from build123d import *

# Parameters (mm, degrees)
F1_DEPTH = 254
F0_W     = 9.525
F0_H     = 9.525
F2_DEPTH = 228.6
F0_W_2   = 114.3
F0_H_2   = 114.3
F3_DEPTH = 177.8
F0_W_3   = 127
F0_H_3   = 127
F4_DEPTH = 127


with BuildPart() as f1:
    # F0 (on Top) → F1 (new body)
    with BuildSketch(Plane.XY):
        Polygon((28.575, 38.1), (-28.575, 38.1), (-28.575, 28.575), (-38.1, 28.575), (-38.1, -28.575), (-28.575, -28.575), (-28.575, -38.1), (28.575, -38.1), (28.575, -28.575), (38.1, -28.575), (38.1, 28.575), (28.575, 28.575), align=None)
    extrude(amount=F1_DEPTH)

    # F0 (on Top) → F2 (join)
    with BuildSketch(Plane.XY):
        Polygon((-38.1, 28.575), (-38.1, 38.1), (-28.575, 38.1), (-28.575, 47.625), (-47.625, 47.625), (-47.625, 28.575), align=None)
        with Locations((-33.3375, 33.3375)):
            Rectangle(F0_W, F0_H)
        Polygon((-38.1, -38.1), (-38.1, -28.575), (-47.625, -28.575), (-47.625, -47.625), (-28.575, -47.625), (-28.575, -38.1), align=None)
        with Locations((-33.3375, -33.3375)):
            Rectangle(F0_W, F0_H)
        Polygon((47.625, -28.575), (38.1, -28.575), (38.1, -38.1), (28.575, -38.1), (28.575, -47.625), (47.625, -47.625), align=None)
        with Locations((33.3375, -33.3375)):
            Rectangle(F0_W, F0_H)
        Polygon((28.575, 47.625), (28.575, 38.1), (38.1, 38.1), (38.1, 28.575), (47.625, 28.575), (47.625, 47.625), align=None)
        with Locations((33.3375, 33.3375)):
            Rectangle(F0_W, F0_H)
    extrude(amount=F2_DEPTH)

    # F0 (on Top) → F3 (join)
    with BuildSketch(Plane.XY):
        Rectangle(F0_W_2, F0_H_2)
        Polygon((-28.575, 47.625), (-28.575, 38.1), (28.575, 38.1), (28.575, 47.625), (47.625, 47.625), (47.625, 28.575), (38.1, 28.575), (38.1, -28.575), (47.625, -28.575), (47.625, -47.625), (28.575, -47.625), (28.575, -38.1), (-28.575, -38.1), (-28.575, -47.625), (-47.625, -47.625), (-47.625, -28.575), (-38.1, -28.575), (-38.1, 28.575), (-47.625, 28.575), (-47.625, 47.625), align=None, mode=Mode.SUBTRACT)
    extrude(amount=F3_DEPTH)

    # F0 (on Top) → F4 (join)
    with BuildSketch(Plane.XY):
        Rectangle(F0_W_3, F0_H_3)
        Rectangle(F0_W_2, F0_H_2, mode=Mode.SUBTRACT)
    extrude(amount=F4_DEPTH)


solid = f1.part
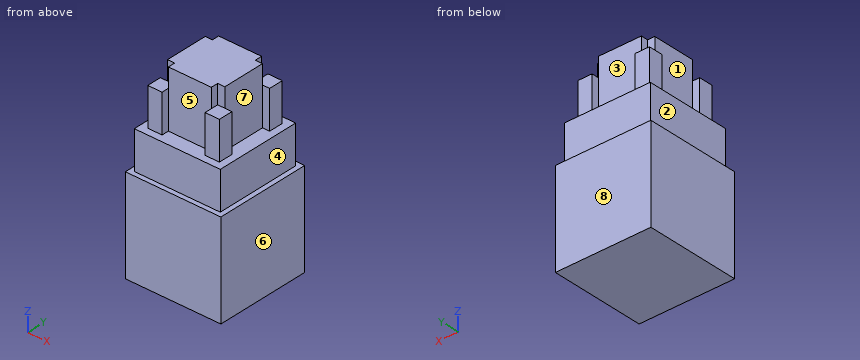
Can you work these out from the model? Positions are in its coordinate system, mm. Face numbers are marked on the shaded views. A direction names the side the tool comes from. Give positions to 0.01 mm unless a question says otherwise; leave off trailing zeros. Order: outer loops, then holes, each group sorted by start corner. A loop starts at its lowest first (then second) coordinate and runs counter-clockwise, first axis right, second up. Notation, with made-up numbers: M -19.5,-3 L 12.5,-3 A4 ccw 12.5,1 Z; hole C -38.5,88.5 d2. An arc over 180 degrees is marked long. Use a Markdown table: item, result. Add a question column.
Item 1: Suppose I cut it at B-B (x = 43). List the corners of the cut face in (y, z) for me (3 decimals), then the cut area to 3 significant figures.
Item 2: Will these pins go through, and if not, where does the flat tip stop? pin 1 (7.5 mm diameter, centred on x = 32.5, z = 241.5, fed in from +Y) (3 decimals); pin 2 (15 mm diameter, centred on x = -36.5, z = 206, fed in from -Y) (3 decimals); pin 3 (5 mm diameter, centred on y = 32, z = 242, fed in from +X) (3 decimals).
Item 3: Suppose I cut it at A-A (y = 21.5). List the corners of the cut face in (x, z) for me, then the cut area to 3 significant figures.
Item 4: If I drill on L1, parallel to X at y = 28, z = 153; L2, parallel to X at y = -8, z = 220; L3, parallel to Z at x = 38, y = -51, over which ranges is the centre line in solid material (lowest first)? Write a range as [from, to].
Item 5: Suppose I cut it at C-C (z = 195). List the corners of the cut face in (x, y) for me (3 decimals), then the cut area to 3 significant figures.
Item 6: We'd pull the mould along Y, two halves only. Please class the marked faces 6, 7 and 8: +Y half, -Y half, draft (parallel to the pull), parting line (faces both ways), or undercut.
Item 7: For the marked faces 1, 2, 3, 4 and 5, which set-ups out of +Z, -Z, +X, -X, +Y, -Y let a thin tool reach every point of the face, with its end or its side?
Item 8: Suppose I cut it at D-D (y = -50.5). List the corners of the cut face in (x, z) for me, then the cut area to 3 significant figures.
Answer sheet:
| question | item | result |
|---|---|---|
| 1 | outline | M -63.5,0 L 63.5,0 L 63.5,127 L 57.15,127 L 57.15,177.8 L 47.625,177.8 L 47.625,228.6 L 28.575,228.6 L 28.575,177.8 L -28.575,177.8 L -28.575,228.6 L -47.625,228.6 L -47.625,177.8 L -57.15,177.8 L -57.15,127 L -63.5,127 Z |
| 1 | area | 23,900 mm² |
| 2 | pin 1 | stops at y = 28.575 |
| 2 | pin 2 | stops at y = -47.625 |
| 2 | pin 3 | stops at x = 28.575 |
| 3 | outline | M -63.5,0 L 63.5,0 L 63.5,127 L 57.15,127 L 57.15,177.8 L 38.1,177.8 L 38.1,254 L -38.1,254 L -38.1,177.8 L -57.15,177.8 L -57.15,127 L -63.5,127 Z |
| 3 | area | 27,700 mm² |
| 4 | L1 | x = [-57.15, 57.15] |
| 4 | L2 | x = [-38.1, 38.1] |
| 4 | L3 | z = [0, 177.8] |
| 5 | outline | M -47.625,-47.625 L -28.575,-47.625 L -28.575,-38.1 L 28.575,-38.1 L 28.575,-47.625 L 47.625,-47.625 L 47.625,-28.575 L 38.1,-28.575 L 38.1,28.575 L 47.625,28.575 L 47.625,47.625 L 28.575,47.625 L 28.575,38.1 L -28.575,38.1 L -28.575,47.625 L -47.625,47.625 L -47.625,28.575 L -38.1,28.575 L -38.1,-28.575 L -47.625,-28.575 Z |
| 5 | area | 6,900 mm² |
| 6 | face 6 | draft |
| 6 | face 7 | undercut |
| 6 | face 8 | +Y half |
| 7 | face 1 | +Z, -X |
| 7 | face 2 | +Z, -X, +Y, -Y |
| 7 | face 3 | +Z, +Y |
| 7 | face 4 | +Z, +X, +Y, -Y |
| 7 | face 5 | +Z, -Y |
| 8 | outline | M -63.5,0 L 63.5,0 L 63.5,127 L 57.15,127 L 57.15,177.8 L -57.15,177.8 L -57.15,127 L -63.5,127 Z |
| 8 | area | 21,900 mm² |
